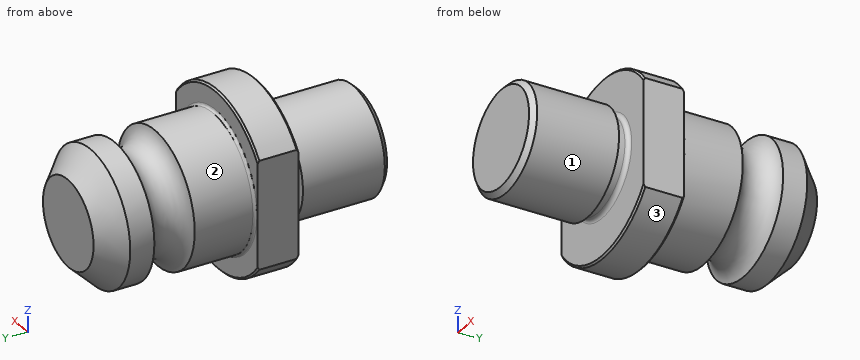
```python
from build123d import *

# Parameters (mm, degrees)
CHAMFER1_SIZE      = 0.508
CHAMFER2_SIZE      = 1.524
CUT_EXTRUDE1_DEPTH = 43.1132
FILLET1_R          = 0.762


with BuildPart() as part:
    # Sketch1 → Revolve1 (revolve)
    with BuildSketch(Plane.XY):
        with BuildLine():
            Line((0, 55.9816), (0, -30.0736))
            Line((0, -30.0736), (-15.875, -30.0736))
            Line((-15.875, -30.0736), (-15.875, -4.318))
            Line((-15.875, -4.318), (-13.6017, -4.318))
            Line((-13.6017, -4.318), (-13.6017, -1.27))
            ThreePointArc((-13.6017, -1.27), (-13.973674388, -0.371974388), (-14.8717, 0))
            Line((-14.8717, 0), (-26.4922, 0))
            Line((-26.4922, 0), (-26.4922, 12.0396))
            Line((-26.4922, 12.0396), (-19.8374, 12.0396))
            Line((-19.8374, 12.0396), (-19.8374, 30.0228))
            ThreePointArc((-19.8374, 30.0228), (-14.859, 35.9918), (-19.8374, 41.9608))
            Line((-19.8374, 41.9608), (-19.8374, 49.0982))
            Line((-19.8374, 49.0982), (-12.954, 55.9816))
            Line((-12.954, 55.9816), (0, 55.9816))
        make_face()
    revolve(axis=Axis((0, -30.0736, 0), (0, -1, 0)))

    # Chamfer1
    chamfer1_edges = [part.edges().sort_by_distance(p)[0] for p in [
        (26.4922, 12.0396, 0),
        (26.4922, 0, 0),
    ]]
    chamfer(chamfer1_edges, length=CHAMFER1_SIZE)

    # Chamfer2
    chamfer2_edges = [part.edges().sort_by_distance(p)[0] for p in [
        (15.875, -30.0736, 0),
    ]]
    chamfer(chamfer2_edges, length=CHAMFER2_SIZE)

    # Sketch2 → Cut-Extrude1 (cut, through all)
    with BuildSketch(Plane(origin=(0, 12.0396, 0), x_dir=(1, 0, 0), z_dir=(0, 1, 0))):
        with BuildLine():
            Line((-20.955, 16.208782676), (-20.955, -16.208782676))
            ThreePointArc((-20.955, -16.208782676), (-26.4922, 0), (-20.955, 16.208782676))
        make_face()
        with BuildLine():
            Line((20.955, 16.208782676), (20.955, -16.208782676))
            ThreePointArc((20.955, -16.208782676), (26.4922, 0), (20.955, 16.208782676))
        make_face()
    extrude(amount=-CUT_EXTRUDE1_DEPTH, mode=Mode.SUBTRACT)

    # Fillet1
    fillet1_edges = [part.edges().sort_by_distance(p)[0] for p in [
        (19.8374, 12.0396, 0),
    ]]
    fillet(fillet1_edges, radius=FILLET1_R)


solid = part.part
```
Geometry check sheet. Reference: the model listing, model coordinates, mm. Face numbers are marked on the shaded views. A direction names the side the tool comes from. Coordinates: 2 decimals unless noted, no trailing zeros. Write each loop counter-clockwise with the first axis right and the second up, starting at its lowest first coordinate (ties: lowest second). Pieces come first, ordered by that corner, then holes. Notation, with made-up numbers: (36, -18.75) -> (92, -18.75) arc R27 ccw to (92, 2.25) -> close; hole circle Ø11 at (44.5, 63). An arc over 180 degrees is marked (long way). Use CSV: the item, a comma, the result in double quotes. Start each with the question number.
Item 1: Thickness scan on line 1 (Z direction, x = -0.5, y = -13.5); line 2 (Y direction, x = 2, z = -20.5); line 3 (Z direction, x = -5.5, y = -10.5). Record the ranges inside material, lowest first.
Item 2: Cross-section at D-D, the plane y = -14. Record the cut outline in (x, z) (3 decimals).
Item 3: Set-up check for the marked faces 1, 2 and 3: record each of +Z, -Z, +X, -X, +Y, -Y from which the full face is reachable in a straight line by a thin tool's end or side.
Item 4: Cross-section at A-A, the plane z = 0. Record the cut outline in (x, y) (3 decimals), plus the area to 3 significant figures.
Item 5: Depth check by flat-ended pin: pin 1 Ø5 at (x, z) = (-14.5, 11) entering from +Y; pin 2 Ø2 at (x, y) = (7.5, 33) entering from -Z; pin 3 Ø10 at (y, z) = (-7, -5) entering from +X (3 decimals). Enter the tip coordinate at first touch or a pass-through.
Item 6: Cross-section at C-C, the plane y = 6.5. Record the cut outline in (x, z) (3 decimals).
Answers:
1,line 1,"-15.87 to 15.87"
1,line 2,"0 to 12.04"
1,line 3,"-14.89 to 14.89"
2,outline,"circle Ø31.75 at (0, 0)"
3,face 1,"-Y"
3,face 2,"+Y"
3,face 3,"-Z, +Y, -Y"
4,outline,"(-20.955, 0) -> (-14.872, 0) arc R1.27 cw to (-13.602, -1.27) -> (-13.602, -4.318) -> (-15.875, -4.318) -> (-15.875, -28.55) -> (-14.351, -30.074) -> (14.351, -30.074) -> (15.875, -28.55) -> (15.875, -4.318) -> (13.602, -4.318) -> (13.602, -1.27) arc R1.27 cw to (14.872, 0) -> (20.955, 0) -> (20.955, 12.04) -> (20.599, 12.04) arc R0.762 cw to (19.837, 12.802) -> (19.837, 30.023) arc R6.068 cw to (19.837, 41.961) -> (19.837, 49.098) -> (12.954, 55.982) -> (-12.954, 55.982) -> (-19.837, 49.098) -> (-19.837, 41.961) arc R6.068 cw to (-19.837, 30.023) -> (-19.837, 12.802) arc R0.762 cw to (-20.599, 12.04) -> (-20.955, 12.04) -> close"
4,area,"3,050 mm^2"
5,pin 1,"y = 53.24"
5,pin 2,"z = -14.66"
5,pin 3,"x = 15.875"
6,outline,"(-20.955, -16.209) arc R26.492 ccw to (20.955, -16.209) -> (20.955, 16.209) arc R26.492 ccw to (-20.955, 16.209) -> close"
